Check sheet for the modelled part. Datum: model origin and axes. Units: mm. Round coordinates to 2 decimals unless told otherwise and drop trailing zeros. Write each loop counter-clockwise with the first axis right and the second up, starting at its lowest first coordinate (ties: lowest second). Pieces come first, ordered by that corner, then holes. Notation, with made-up numbers: M -40,26.25 L -36,26.25 A25 ccw -36,63.25 Z; hole C -2,32.25 d5. An arc over 180 degrees is marked long. Answer in a Markdown table with one row per item.
Autodesk Inventor part; units mm, degrees
ref_plane "YZ Plane" through (0, 0, 0) normal (1, 0, 0) x (0, 1, 0)
ref_plane "XZ Plane" through (0, 0, 0) normal (0, 1, 0) x (-1, 0, 0)
ref_plane "XY Plane" through (0, 0, 0) normal (0, 0, 1) x (1, 0, 0)
sketch "Sketch1" plane through (0, 0, 0) normal (0, 1, 0) x (-1, 0, 0)
  circle A0 centre (0, 0) radius 85
  line L0 (7.5, 84.6685) -> (7.5, -84.6685)
  dimension "d0" = 170
  dimension "d1" = 7.5
extrude "Extrusion1" add sketch "Sketch1" along normal blind 3 contours A0 L0 picked at (34.1822, 19.1304)
sketch "Sketch2" plane through (0, 3, 0) normal (0, 1, 0) x (1, 0, 0)
  line L0 (-20, 55) -> (-58, 55) construction
  line L1 (-58, 55) -> (-58, -55) construction
  line L2 (-58, -55) -> (-20, -55) construction
  line L3 (-20, -55) -> (-20, 55) construction
  line L4 (-20, 40) -> (-17, 40)
  line L5 (-17, 40) -> (-17, 20)
  line L6 (-17, 20) -> (-20, 20)
  line L7 (-20, 20) -> (-20, 40)
  line L8 (-20, 55) -> (-58, 55)
  line L9 (-58, 55) -> (-58, -55)
  line L10 (-58, -55) -> (-20, -55)
  line L11 (-20, -55) -> (-20, 55)
  line L12 (-20, -20) -> (-17, -20)
  line L13 (-17, -20) -> (-17, -40)
  line L14 (-17, -40) -> (-20, -40)
  line L15 (-20, -40) -> (-20, -20)
  line L16 (-58, 40) -> (-61, 40)
  line L17 (-61, 40) -> (-61, 20)
  line L18 (-61, 20) -> (-58, 20)
  line L19 (-58, 20) -> (-58, 40)
  line L20 (-58, -20) -> (-61, -20)
  line L21 (-61, -20) -> (-61, -40)
  line L22 (-61, -40) -> (-58, -40)
  line L23 (-58, -40) -> (-58, -20)
  line L24 (-34, 55) -> (-44, 55)
  line L25 (-44, 55) -> (-44, 58)
  line L26 (-44, 58) -> (-34, 58)
  line L27 (-34, 58) -> (-34, 55)
  line L28 (-34, -55) -> (-44, -55)
  line L29 (-44, -55) -> (-44, -58)
  line L30 (-44, -58) -> (-34, -58)
  line L31 (-34, -58) -> (-34, -55)
  point P0 (0, 0)
  point P1 (-20, 0)
  point P2 (-39, 58)
  point P3 (-39, 55)
  dimension "d4" = 38
  dimension "d5" = 110
  dimension "d6" = 20
  dimension "d7" = 3
  dimension "d8" = 20
  dimension "d9" = 20
  dimension "d10" = 3
  dimension "d11" = 20
  dimension "d12" = 20
  dimension "d13" = 3
  dimension "d14" = 10
  dimension "d15" = 3
  dimension "d16" = 10
  dimension "d17" = 3
extrude "Extrusion2" cut sketch "Sketch2" against normal blind 3
sketch "Sketch3" plane through (0, 3, 0) normal (0, 1, 0) x (1, 0, 0)
  line L0 (-66, 1.5) -> (-76, 1.5)
  line L1 (-76, 1.5) -> (-76, -1.5)
  line L2 (-76, -1.5) -> (-66, -1.5)
  line L3 (-66, -1.5) -> (-66, 1.5)
  line L4 (-61, 20) -> (-61, 40)
  line L5 (-58, -20) -> (-58, 20)
  point P0 (0, 0)
  point P1 (-66, 0)
  point P2 (-58, 0)
  dimension "d20" = 10
  dimension "d21" = 3
  dimension "d22" = 5
extrude "Extrusion3" cut sketch "Sketch3" against normal blind 3
sketch "Sketch4" plane through (0, 3, 0) normal (0, 1, 0) x (1, 0, 0)
  line L0 (-7.5, -84.6685) -> (-7.5, 84.6685)
  line L1 (-7.5, 75) -> (-25, 75)
  line L2 (-25, 75) -> (-25, 60)
  line L3 (-25, 60) -> (-7.5, 60)
  line L4 (-7.5, 60) -> (-7.5, 75)
  point P0 (0, 0)
  dimension "d25" = 25
  dimension "d26" = 60
  dimension "d27" = 15
extrude "Extrusion4" cut sketch "Sketch4" against normal blind 3
mirror "Mirror1" about plane through (0, 0, 0) normal (0, 0, 1) of "Extrusion4"
sketch "Sketch5" plane through (0, 3, 0) normal (0, 1, 0) x (1, 0, 0)
  point P0 (0, 0)
properties part number "Mid Plate"
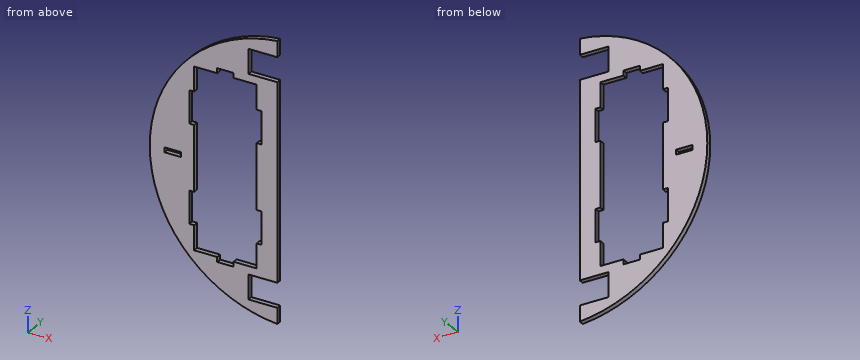
1. Section check A-A, the plane x = -11.5. Record the cut outline in (y, z).
Found:
| item | result |
|---|---|
| outline | M 0,-84.22 L 3,-84.22 L 3,-75 L 0,-75 Z; M 0,-60 L 3,-60 L 3,60 L 0,60 Z; M 0,75 L 3,75 L 3,84.22 L 0,84.22 Z |
2. Scan lines: L1, parallel to X at y = 1.7, z = 54; L2, parallel to X at y = 0.8, z = -38; L3, parallel to Z at x = -23, y = 1.1. Record each from-to range of solid material in increasing order.
Found:
| item | result |
|---|---|
| L1 | x = -65.64 to -58, -20 to -7.5 |
| L2 | x = -76.03 to -61, -17 to -7.5 |
| L3 | z = -81.83 to -75, -60 to -55, 55 to 60, 75 to 81.83 |
3. Section check B-B, the plane z = 27. Record the cut outline in (x, y).
Found:
| item | result |
|---|---|
| outline | M -80.6,0 L -61,0 L -61,3 L -80.6,3 Z; M -17,0 L -7.5,0 L -7.5,3 L -17,3 Z |
4. Go/stop test with flat-tipped pins: pin 1 (1.5 mm diameter, centred on x = -75, y = 2.5, fed in from +Z); pin 2 (1.5 mm diameter, centred on x = -59.5, y = 1.5, fed in from -Z); pin 3 (1.5 mm diameter, centred on x = -20.5, y = 1.5, fed in from -Z). Record where each tip stops, or that it passes through.
Found:
| item | result |
|---|---|
| pin 1 | stops at z = 41.38 |
| pin 2 | stops at z = -61.43 |
| pin 3 | stops at z = -82.67 |
5. Section check D-D, the plane y = 1. Count the separate pieces of the cut face and the enclosed holes in it, and give its area (3 significant figures).
Found:
| item | result |
|---|---|
| separate pieces | 1 |
| enclosed holes | 2 |
| area | 5,040 mm2 |
6. Section check C-C, the plane x = -26.5. Record the cut outline in (y, z), and give its area (3 significant figures).
Found:
| item | result |
|---|---|
| outline | M 0,-80.76 L 3,-80.76 L 3,-55 L 0,-55 Z; M 0,55 L 3,55 L 3,80.76 L 0,80.76 Z |
| area | 155 mm2 |
